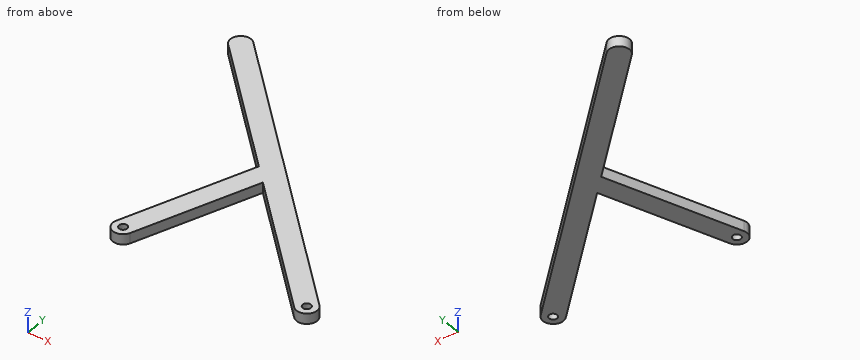
from build123d import *

# Parameters (mm, degrees)
BOSS_EXTRUDE1_DEPTH = 10
SKETCH2_R           = 4
CUT_EXTRUDE1_DEPTH  = 10


# Read off the part's stored shape, not the designer's step: Boss-Extrude1
with BuildPart() as part:
    # Boss-Extrude1 outline → Boss-Extrude1 (new body)
    with BuildSketch(Plane.XY):
        with BuildLine():
            ThreePointArc((-7.071067812, -7.071067812), (7.071067812, -7.071067812), (7.071067812, 7.071067812))
            Line((7.071067812, 7.071067812), (-247.487373415, 261.629509039))
            ThreePointArc((-247.487373415, 261.629509039), (-261.629509039, 261.629509039), (-261.629509039, 247.487373415))
            Line((-261.629509039, 247.487373415), (-143.543524061, 129.401388437))
            Line((-143.543524061, 129.401388437), (-189.396926208, 3.420201433))
            ThreePointArc((-189.396926208, 3.420201433), (-183.420201433, -9.396926208), (-170.603073792, -3.420201433))
            Line((-170.603073792, -3.420201433), (-127.939403887, 113.797268263))
            Line((-127.939403887, 113.797268263), (-7.071067812, -7.071067812))
        make_face()
    extrude(amount=BOSS_EXTRUDE1_DEPTH)

    # Sketch2 → Cut-Extrude1 (cut)
    with BuildSketch(Plane.XY.offset(10)):
        Circle(SKETCH2_R)
        with Locations((-180, 0)):
            Circle(SKETCH2_R)
    extrude(amount=-CUT_EXTRUDE1_DEPTH, mode=Mode.SUBTRACT)


solid = part.part
Build history of the part. All positions in model axes, mm. Give positions to 0.01 mm unless a question says otherwise; leave off trailing zeros. Order: outer loops, then holes, each group sorted by start corner. A loop starts at its lowest first (then second) coordinate and runs counter-clockwise, first axis right, second up. Notation, with made-up numbers: M 17.5,9 L 35.5,9 A13 cw 35.5,17 Z; hole C 87,-26.75 d10. An arc over 180 degrees is marked long. Use one line per item in the form item = value.
1) Saw through at C-C (z = 8). Give the cut face in (x, y).
Calculated:
outline = M -261.63,247.49 L -143.54,129.4 L -189.4,3.42 A10 ccw -170.6,-3.42 L -127.94,113.8 L -7.07,-7.07 A10 ccw 7.07,7.07 L -247.49,261.63 A10 ccw Z; hole C -180,0 d8; hole C 0,0 d8
2) Saw through at A-A (y = 0). Give the cut face in (x, z), plus the area to 3 significant figures.
Calculated:
outline = M -190,0 L -184,0 L -184,10 L -190,10 Z; M -176,0 L -169.36,0 L -169.36,10 L -176,10 Z; M -14.14,0 L -4,0 L -4,10 L -14.14,10 Z; M 4,0 L 10,0 L 10,10 L 4,10 Z
area = 288 mm2
3) Saw through at D-D (y = 27.5). Give the cut face in (x, z).
Calculated:
outline = M -180.63,0 L -159.35,0 L -159.35,10 L -180.63,10 Z; M -41.64,0 L -13.36,0 L -13.36,10 L -41.64,10 Z
4) Drop flat-ended pins along their axis: pin 1 (4 mm diameter, centred on x = -62.5, z = 7.5, fed in from +Y); pin 2 (1.5 mm diameter, centred on y = 38.5, z = 7, fed in from +X); pin 3 (2 mm diameter, centred on y = 146.5, z = 5, fed in from -X). Give the stop position or say it passes through.
Calculated:
pin_1 = 78.64
pin_2 = -23.61
pin_3 = -161.64
5) Saw through at B-B (x = -153). Give the cut face in (y, z), plus the area to 3 significant figures.
Calculated:
outline = M 44.94,0 L 103.42,0 L 103.42,10 L 44.94,10 Z; M 138.86,0 L 167.14,0 L 167.14,10 L 138.86,10 Z
area = 868 mm2
6) Probe probe 1 along X at (y, z) = (80, 3.5); probe 2 along X at (y, z) = (66, 6.25); probe 3 along Y at (x, z) = (0, 6). List the from-to ranges inside material, lowest first.
Calculated:
probe_1 = -161.52 to -140.24, -94.14 to -65.86
probe_2 = -166.62 to -145.34, -80.14 to -51.86
probe_3 = -10 to -4, 4 to 14.14
